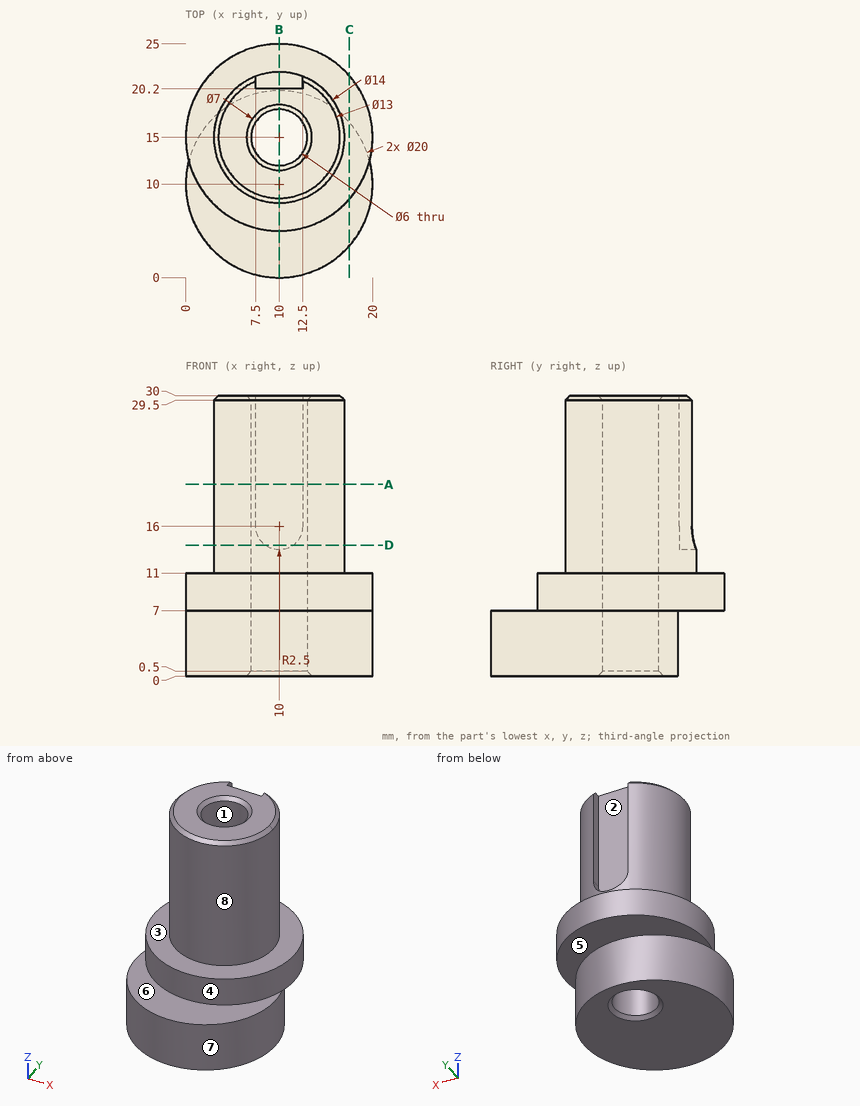
Verification items for this drawing (mm, ordinates from the low corner). A direction names the side the tool comes from. Round coordinates to 2 decimals unless told otherwise and drop trailing zeros. Order: outer loops, then holes, each group sorted by start corner. A loop starts at its lowest first (then second) coordinate and runs counter-clockwise, first axis right, second up. Notation, with made-up numbers: M 76,-27.75 L 93,-27.75 A6 cw 93,-16.75 Z; hole C 44,13 d6. An arc over 180 degrees is marked long. Answer in a Markdown table with one row per item. Add a question column.
Item 1: Material ranges on L1, parallel to Y at x = 10, z = 6.5; L2, parallel to Y at x = 10, z = 23.5; L3, parallel to Z at x = 17.25, y = 21, recorded low to high. Write a range as [from, to].
Item 2: Set-up check for the marked faces 5, 6, 7 and 8: record each of +Z, -Z, +X, -X, +Y, -Y from which the full face is reachable in a straight line by a thin tool's end or side.
Item 3: Depth check by flat-ended pin: pin 1 Ø8 at (x, z) = (5, 16.5) entering from -Y; pin 2 Ø12 at (y, z) = (14, 21) entering from -X; pin 3 Ø6 at (x, z) = (15, 21.5) entering from -Y. Enter the tip coordinate at first touch or a pass-through.
Item 4: Sectioned sample at B-B, the plane x = 10. Enter the section's corners in (y, z), plus the area to 3 significant figures.
Item 5: Sectioned sample at C-C, the plane x = 17.5. Enter the section's corners in (y, z).
Item 6: Sectioned sample at A-A, the plane z = 20.5. Enter the section's corners in (x, y).
Item 7: Draft check along X on the marked faces 1, 2, 3 and 4. Enter one of: released by +X, released by -X, zero draft, split by the parting line, or undercut.
Item 8: Sectioned sample at D-D, the plane z = 14. Enter the section's corners in (x, y).
Filled in:
| question | item | result |
|---|---|---|
| 1 | L1 | y = [0, 12], [18, 20] |
| 1 | L2 | y = [8, 12], [18, 20.2] |
| 1 | L3 | z = [7, 11] |
| 2 | face 5 | -Z, +Y |
| 2 | face 6 | +Z, -Y |
| 2 | face 7 | -Z |
| 2 | face 8 | +Z |
| 3 | pin 1 | stops at y = 8.07 |
| 3 | pin 2 | stops at x = 3 |
| 3 | pin 3 | stops at y = 8.29 |
| 4 | outline | M 0,0 L 11.5,0 L 12,0.5 L 12,29.5 L 11.5,30 L 8.5,30 L 8,29.5 L 8,11 L 5,11 L 5,7 L 0,7 Z; M 18,0.5 L 18.5,0 L 20,0 L 20,7 L 25,7 L 25,11 L 22,11 L 22,13.5 L 20.2,13.5 L 20.2,30 L 18.5,30 L 18,29.5 Z |
| 4 | area | 276 mm² |
| 5 | outline | M 3.39,0 L 16.61,0 L 16.61,7 L 21.61,7 L 21.61,11 L 8.39,11 L 8.39,7 L 3.39,7 Z |
| 6 | outline | M 7.5,20.2 L 7.5,21.54 A7 ccw long 12.5,21.54 L 12.5,20.2 Z; hole C 10,15 d6 |
| 7 | face 1 | undercut |
| 7 | face 2 | undercut |
| 7 | face 3 | zero draft |
| 7 | face 4 | split by the parting line |
| 8 | outline | M 8.5,20.2 L 8.5,21.84 A7 ccw long 11.5,21.84 L 11.5,20.2 Z; hole C 10,15 d6 |
